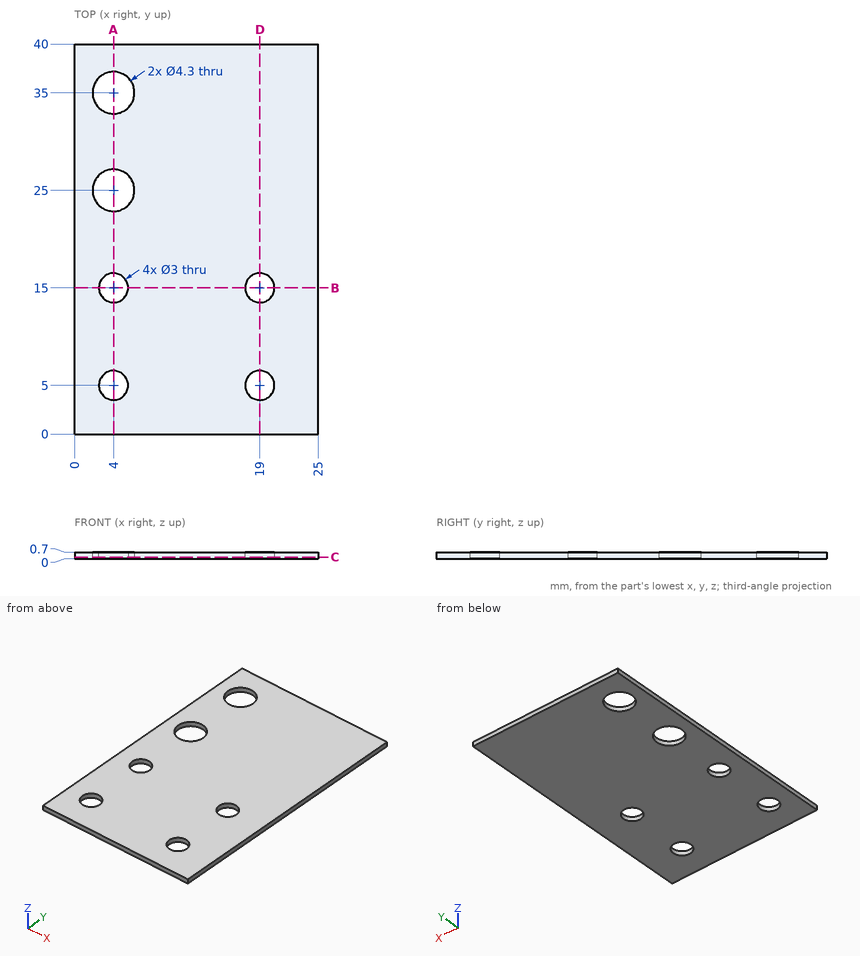
Part print with two shaded views. Sizes in mm from the minimum x, y, z corner. Coordinates: 2 decimals unless noted, no trailing zeros. Loops run counter-clockwise (first coordinate to the right, second up) from the corner with the lowest first, then second, coordinate; pieces in that order, holes last. Notation, with made-up numbers: M -15,88.25 L 38,88.25 A18 cw 38,102.25 Z; hole C 71,45 d10. An arc over 180 degrees is marked long. Use CSV: the item, a comma, the result in double quotes. Start each with the question number.
1. Band-saw the part on D-D, the plane x = 19. List the corners of the cut face in (y, z).
2. Band-saw the part on B-B, the plane y = 15. List the corners of the cut face in (x, z).
3. Band-saw the part on C-C, the plane z = 0.2. List the corners of the cut face in (x, y).
4. Flat gauge pin, fed straight in: pin 1 (3 mm diameter, centred on x = 18.5, y = 13.5, fed in from -Z). Where does the tip first touch, or does it go through?
5. Probe probe 1 along Y at (x, z) = (19, 0.4); probe 2 along Y at (x, z) = (4, 0.55); probe 3 along Y at (x, z) = (5.75, 0.65). List the from-to ranges inside material, lowest first. Write a range as [from, to].
6. Band-saw the part on A-A, the plane x = 4. List the corners of the cut face in (y, z), then the cut area to 3 significant figures.
Entries:
1,outline,"M 0,0 L 3.5,0 L 3.5,0.7 L 0,0.7 Z; M 6.5,0 L 13.5,0 L 13.5,0.7 L 6.5,0.7 Z; M 16.5,0 L 40,0 L 40,0.7 L 16.5,0.7 Z"
2,outline,"M 0,0 L 2.5,0 L 2.5,0.7 L 0,0.7 Z; M 5.5,0 L 17.5,0 L 17.5,0.7 L 5.5,0.7 Z; M 20.5,0 L 25,0 L 25,0.7 L 20.5,0.7 Z"
3,outline,"M 0,0 L 25,0 L 25,40 L 0,40 Z; hole C 4,25 d4.3; hole C 4,35 d4.3; hole C 4,5 d3; hole C 4,15 d3; hole C 19,5 d3; hole C 19,15 d3"
4,pin 1,"stops at z = 0"
5,probe 1,"y = [0, 3.5], [6.5, 13.5], [16.5, 40]"
5,probe 2,"y = [0, 3.5], [6.5, 13.5], [16.5, 22.85], [27.15, 32.85], [37.15, 40]"
5,probe 3,"y = [0, 23.75], [26.25, 33.75], [36.25, 40]"
6,outline,"M 0,0 L 3.5,0 L 3.5,0.7 L 0,0.7 Z; M 6.5,0 L 13.5,0 L 13.5,0.7 L 6.5,0.7 Z; M 16.5,0 L 22.85,0 L 22.85,0.7 L 16.5,0.7 Z; M 27.15,0 L 32.85,0 L 32.85,0.7 L 27.15,0.7 Z; M 37.15,0 L 40,0 L 40,0.7 L 37.15,0.7 Z"
6,area,"17.8 mm2"
